The listing builds one solid part. Answer for the finished solid, in the listing's coordinates (mm). A direction names the side the tool comes from. Give positions to 0.01 mm unless a question says otherwise; leave off trailing zeros. Write each loop counter-clockwise with the first axis right and the second up, starting at its lowest first coordinate (ties: lowest second). Pieces come first, ordered by that corner, then holes. Notation, with made-up numbers: (46, 27.25) - (80, 27.25) arc R3 ccw to (80, 32.25) - close; hole circle Ø10 at (-7, -26.75). An arc over 180 degrees is marked (long way). Answer as CSV lines item,"result". Start each with the question number.
(1) Each of these flat-tipped pins is pushed along its axis until it touches: pin 1 Ø7.5 at (x, y) = (51.08, 54.58) entering from -Z; pin 2 Ø8 at (x, z) = (25, -55) entering from +Y; pin 3 Ø1 at (x, y) = (24.5, 49.5) entering from +Z (3 decimals); pin 4 Ø7.5 at (x, z) = (19.05, -19.05) entering from +Y (3 decimals). Where does it stop, or does it pass through?
(2) For a pull along Z with two mould halves and no side action, classify faces 1 (the face through (24, 30, -63.5)), 2 (the face through (19.775, 1.565, -16.748)), 3 (the face through (56.208, 27.244, -61.935)) as pulls with the +Z half, pulls with the -Z half, needs draft (parallel to the pull), parting line crosses it, or undercut.
(3) For faces 4 (the face through (31, 3.175, -29)), 5 (the face through (46.485, 1.565, -17.753)), determine the directions among +Z, -Z, +X, -X, +Y, -Y from which every point of the face is accessible in a straight line to the end or side of a thin tool.
(4) Find section B-B (x = 44.45). Write down the section's boundary in (y, z) (3 decimals).
(5) Find section D-D (x = 8). Write down the section's boundary in (y, z) (3 decimals), then the cut area to 3 significant figures.
(6) Find section A-A (y = 38.1). Write down the section's boundary in (x, z) (3 decimals), then the cut area to 3 significant figures.
(7) Straight lines are drawn through the part: probe 1 along X at (y, z) = (1, -19); probe 2 along Y at (x, z) = (43.5, -10.5) (3 decimals); probe 3 along Z at (x, y) = (25, 14) (3 decimals). For each, find the intervals that lie inside material, in ascending order.
(8) Find section C-C (z = -19.05). Write down the section's boundary in (x, y) (3 decimals), then the cut area to 3 significant figures.
from build123d import *

# Parameters (mm, degrees)
SKETCH1_W              = 63.5
SKETCH1_H              = 63.5
SKETCH1_R              = 2.413
BOSS_EXTRUDE1_DEPTH    = 3.175
SKETCH2_W              = 63.5
SKETCH2_H              = 3.175
BOSS_EXTRUDE2_DEPTH    = 66.675
SKETCH3_R              = 10.16
SKETCH3_R_2            = 2.413
CUT_EXTRUDE2_DEPTH     = 60.325
FILLET1_R              = 2.54
CONVERT_SOLID1_DEPTH   = 63.5
CONVERT_SOLID1_2_DEPTH = 63.5


# Read off the part's stored shape, not the designer's step: Convert-Solid1
with BuildPart() as part:
    # Sketch1 → Boss-Extrude1 (new body)
    with BuildSketch(Plane(origin=(0, 0, 0), x_dir=(1, 0, 0), z_dir=(0, 1, 0))):
        with Locations((31.75, 31.75)):
            Rectangle(SKETCH1_W, SKETCH1_H)
        with Locations(Location((19.05, 44.45, 0), (0, 0, 270))):
            Circle(SKETCH1_R, mode=Mode.SUBTRACT)
        with Locations(Location((44.45, 44.45, 0), (0, 0, 270))):
            Circle(SKETCH1_R, mode=Mode.SUBTRACT)
        with Locations(Location((19.05, 19.05, 0), (0, 0, 270))):
            Circle(SKETCH1_R, mode=Mode.SUBTRACT)
        with Locations(Location((44.45, 19.05, 0), (0, 0, 270))):
            Circle(SKETCH1_R, mode=Mode.SUBTRACT)
    extrude(amount=BOSS_EXTRUDE1_DEPTH)

    # Sketch2 → Boss-Extrude2 (add)
    with BuildSketch(Plane(origin=(0, 3.175, 0), x_dir=(1, 0, 0), z_dir=(0, 1, 0))):
        with Locations((31.75, 61.9125)):
            Rectangle(SKETCH2_W, SKETCH2_H)
    extrude(amount=BOSS_EXTRUDE2_DEPTH)

    # Sketch3 → Cut-Extrude2 (cut)
    with BuildSketch(Plane(origin=(0, 0, -63.5), x_dir=(-1, 0, 0), z_dir=(0, 0, -1))):
        with Locations((-31.75, 38.1)):
            Circle(SKETCH3_R)
        with Locations((-27.144154857, 63.078914919)):
            Circle(SKETCH3_R_2)
        with Locations((-7.81470255, 46.600678559)):
            Circle(SKETCH3_R_2)
        with Locations((-12.420547693, 21.621763641)):
            Circle(SKETCH3_R_2)
        with Locations((-36.355845143, 13.121085081)):
            Circle(SKETCH3_R_2)
        with Locations((-55.68529745, 29.599321441)):
            Circle(SKETCH3_R_2)
        with Locations((-51.079452307, 54.578236359)):
            Circle(SKETCH3_R_2)
    extrude(amount=-CUT_EXTRUDE2_DEPTH, mode=Mode.SUBTRACT)

    # Fillet1
    fillet1_edges = [part.edges().sort_by_distance(p)[0] for p in [
        (0, 69.85, -61.9125),
        (63.5, 69.85, -61.9125),
        (63.5, 1.5875, 0),
        (0, 1.5875, 0),
    ]]
    fillet(fillet1_edges, radius=FILLET1_R)

    # Convert-Solid1 outline → Convert-Solid1 (cut)
    with BuildSketch(Plane.YZ):
        with BuildLine():
            Line((0, -63.5), (5.555000066, -63.5))
            ThreePointArc((5.555000066, -63.5), (1.62702185, -61.87297815), (0, -57.944999934))
            Line((0, -57.944999934), (0, -63.5))
        make_face()
    extrude(amount=CONVERT_SOLID1_DEPTH, mode=Mode.SUBTRACT)

    # Convert-Solid1 2 outline → Convert-Solid1 2 (add)
    with BuildSketch(Plane.YZ):
        with BuildLine():
            Line((3.175, -60.325), (5.555000066, -60.325))
            ThreePointArc((5.555000066, -60.325), (3.87208588, -59.62791412), (3.175, -57.944999934))
            Line((3.175, -57.944999934), (3.175, -60.325))
        make_face()
    extrude(amount=CONVERT_SOLID1_2_DEPTH)


solid = part.part
Result set:
1,pin 1,"z = -63.5"
1,pin 2,"y = 3.42"
1,pin 3,"z = -60.325"
1,pin 4,"y = 3.175"
2,face 1,"pulls with the -Z half"
2,face 2,"undercut"
2,face 3,"needs draft"
3,face 4,"+Z, +X, -X, +Y"
3,face 5,"+Y, -Y"
4,outline,"(0, -57.945) arc R5.555 ccw to (5.555, -63.5) - (69.85, -63.5) - (69.85, -60.325) - (5.555, -60.325) arc R2.38 cw to (3.175, -57.945) - (3.175, -46.863) - (0, -46.863) - close; (0, -42.037) - (3.175, -42.037) - (3.175, -21.463) - (0, -21.463) - close; (0, -16.637) - (3.175, -16.637) - (3.175, 0) - (0, 0) - close"
5,outline,"(0, -57.945) arc R5.555 ccw to (5.555, -63.5) - (44.195, -63.5) - (44.195, -60.325) - (5.555, -60.325) arc R2.38 cw to (3.175, -57.945) - (3.175, 0) - (0, 0) - close; (49.007, -63.5) - (69.85, -63.5) - (69.85, -60.325) - (49.007, -60.325) - close"
5,area,"393 mm^2"
6,outline,"(0, -63.5) - (21.59, -63.5) - (21.59, -60.325) - (0, -60.325) - close; (41.91, -63.5) - (63.5, -63.5) - (63.5, -60.325) - (41.91, -60.325) - close"
6,area,"137 mm^2"
7,probe 1,"0 to 16.64, 21.46 to 42.04, 46.86 to 63.5"
7,probe 2,"0 to 3.175"
7,probe 3,"-63.5 to -60.325"
8,outline,"(0, 0) - (16.637, 0) - (16.637, 3.175) - (0, 3.175) - close; (21.463, 0) - (42.037, 0) - (42.037, 3.175) - (21.463, 3.175) - close; (46.863, 0) - (63.5, 0) - (63.5, 3.175) - (46.863, 3.175) - close"
8,area,"171 mm^2"
